Read the model definition and answer for the solid it produces. Units are mm, in the model's axes. A direction names the side the tool comes from. Coordinates: 2 decimals unless noted, no trailing zeros. Loops run counter-clockwise (first coordinate to the right, second up) from the corner with the lowest first, then second, coordinate; pieces in that order, holes last.
from build123d import *

# Parameters (mm, degrees)
F0_W      = 108
F0_H      = 130
F1_DEPTH  = 51.5
F2_R      = 6.5
F3_DEPTH  = 51.501
F4_R      = 10
F5_DEPTH  = 20
F7_R      = 32
F8_DEPTH  = 18.5
F10_DEPTH = 8
F11_R     = 10
F12_DEPTH = 78.001
F13_SIZE  = 13
F14_W     = 20
F14_H     = 55
F14_H_2   = 20
F14_W_2   = 44
F15_DEPTH = 5


with BuildPart() as f1:
    # F0 (on Right) → F1 (new body)
    with BuildSketch(Plane.YZ):
        Rectangle(F0_W, F0_H)
    extrude(amount=-F1_DEPTH)

    # F2 (on face) → F3 (cut, through all)
    with BuildSketch(Plane(origin=(-51.5, 0, 0), x_dir=(0, -1, 0), z_dir=(-1, 0, 0))):
        with Locations((42, 47)):
            Circle(F2_R)
        with Locations((-42, 47)):
            Circle(F2_R)
        with Locations((-42, -47)):
            Circle(F2_R)
        with Locations((42, -47)):
            Circle(F2_R)
    extrude(amount=-F3_DEPTH, mode=Mode.SUBTRACT)

    # F4 (on face) → F5 (cut)
    with BuildSketch(Plane(origin=(-51.5, 0, 0), x_dir=(0, -1, 0), z_dir=(-1, 0, 0))):
        with Locations((-42, 47)):
            Circle(F4_R)
        with Locations((-42, -47)):
            Circle(F4_R)
        with Locations((42, 47)):
            Circle(F4_R)
        with Locations((42, -47)):
            Circle(F4_R)
    extrude(amount=-F5_DEPTH, mode=Mode.SUBTRACT)

    # F7 (on offset) → F8 (join, through all)
    with BuildSketch(Plane.YZ.offset(-70)):
        Circle(F7_R)
    extrude(amount=F8_DEPTH)

    # F9 (on face) → F10 (join)
    with BuildSketch(Plane(origin=(-70, 0, 0), x_dir=(0, -1, 0), z_dir=(-1, 0, 0))):
        Polygon((23.6713610368, 0), (11.8356805184, 20.5), (-11.8356805184, 20.5), (-23.6713610368, 0), (-11.8356805184, -20.5), (11.8356805184, -20.5), align=None)
    extrude(amount=F10_DEPTH)

    # F11 (on face) → F12 (cut, through all)
    with BuildSketch(Plane(origin=(-78, 0, 0), x_dir=(0, -1, 0), z_dir=(-1, 0, 0))):
        Circle(F11_R)
    extrude(amount=-F12_DEPTH, mode=Mode.SUBTRACT)

    # F13
    f13_edges = [f1.edges().sort_by_distance(p)[0] for p in [
        (-25.75, -54, 65),
        (-25.75, 54, 65),
        (-25.75, -54, -65),
        (-25.75, 54, -65),
    ]]
    chamfer(f13_edges, length=F13_SIZE)

    # F14 (on face) → F15 (cut)
    with BuildSketch(Plane.YZ):
        with Locations((0, 37.5)):
            Rectangle(F14_W, F14_H)
        Rectangle(F14_W, F14_H_2)
        with Locations((-32, 0)):
            Rectangle(F14_W_2, F14_H_2)
        with Locations((32, 0)):
            Rectangle(F14_W_2, F14_H_2)
        with Locations((0, -37.5)):
            Rectangle(F14_W, F14_H)
    extrude(amount=-F15_DEPTH, mode=Mode.SUBTRACT)


solid = f1.part
Item 1: A cutting plane is placed at B-B on z = -47. Determine the outline of the cut face in (x, y), then the cut area to 3 significant figures.
Numbers:
outline: (-51.5, -54) - (0, -54) - (0, -48.5) - (-31.5, -48.5) - (-31.5, -52) - (-51.5, -52) - close; (-51.5, -32) - (-31.5, -32) - (-31.5, -35.5) - (0, -35.5) - (0, -10) - (-5, -10) - (-5, 10) - (0, 10) - (0, 35.5) - (-31.5, 35.5) - (-31.5, 32) - (-51.5, 32) - close; (-51.5, 52) - (-31.5, 52) - (-31.5, 48.5) - (0, 48.5) - (0, 54) - (-51.5, 54) - close
area: 3,840 mm2
Item 2: Determine the mould class of faces 5 (the face through (-73.944, 17.836, -10.107)), 6 (the face through (-2, 10, 37)), 7 (the face through (-15.971, 47.158, -50.955)) for opening direction Z: released by +Z, released by -Z, zero draft, split by the parting line, or undercut.
Numbers:
face 5: released by -Z
face 6: zero draft
face 7: undercut
Item 3: A cutting plane is placed at C-C on y = 0. Determine the outline of the cut face in (x, z).
Numbers:
outline: (-78, -20.5) - (-70, -20.5) - (-70, -32) - (-51.5, -32) - (-51.5, -65) - (-5, -65) - (-5, -10) - (-78, -10) - close; (-78, 10) - (-5, 10) - (-5, 65) - (-51.5, 65) - (-51.5, 32) - (-70, 32) - (-70, 20.5) - (-78, 20.5) - close
Item 4: A cutting plane is placed at A-A on x = -48. Determine the outline of the cut face in (y, z), then the cut area to 3 significant figures.
Numbers:
outline: (-54, -52) - (-41, -65) - (41, -65) - (54, -52) - (54, 52) - (41, 65) - (-41, 65) - (-54, 52) - close; hole circle Ø20 at (-42, -47); hole circle Ø20 at (-42, 47); hole circle Ø20 at (0, 0); hole circle Ø20 at (42, -47); hole circle Ø20 at (42, 47)
area: 12,100 mm2
Item 5: Which of the six approach directions +Z, -Z, +X, -X, +Y, -Y give full straight-line access (tool end or side, diameter ignored) to faces 1 (the face through (-2, 10, -38)), 2 (the face through (-41.64, 44.17, 37.24)), 3 (the face through (-2, 32, -10)), 4 (the face through (-73.944, -17.671, -10.393))?
Numbers:
face 1: +Z, -Z, +X
face 2: -X
face 3: +X, +Y, -Y
face 4: -Z, -X, -Y
Item 6: A cutting plane is placed at D-D on y = -21. Determine the outline of the cut face in (x, z), then the cut area to 3 significant figures.
Numbers:
outline: (-78, -4.63) - (-70, -4.63) - (-70, -24.15) - (-51.5, -24.15) - (-51.5, -65) - (0, -65) - (0, -10) - (-5, -10) - (-5, 10) - (0, 10) - (0, 65) - (-51.5, 65) - (-51.5, 24.15) - (-70, 24.15) - (-70, 4.63) - (-78, 4.63) - close
area: 7,560 mm2
Item 7: Given pin 1 (10 mm diameter, centred on y = 40, z = 44.5, fed in from -X); pin 2 (10 mm diameter, centred on x = -57, y = -43, fed in from -Z); pin 3 (21 mm diameter, centred on y = 42, z = 47, fed in from -X), each flat-ended and moving along its own axis, determine where each tip first touches the part or whether it passes through.
Numbers:
pin 1: stops at x = -31.5
pin 2: passes through
pin 3: stops at x = -51.5
Item 8: Find the intervals of material crossed by line 1 along Y through (x, z) = (-41, -52); line 2 along Z through (x, y) = (-25.5, -48); line 3 along Y through (x, z) = (-51, 54), in increasing order.
Numbers:
line 1: y = -54 to -50.66, -33.34 to 33.34, 50.66 to 54
line 2: z = -58 to -49.5, -44.5 to 44.5, 49.5 to 58
line 3: y = -52 to -49.14, -34.86 to 34.86, 49.14 to 52
